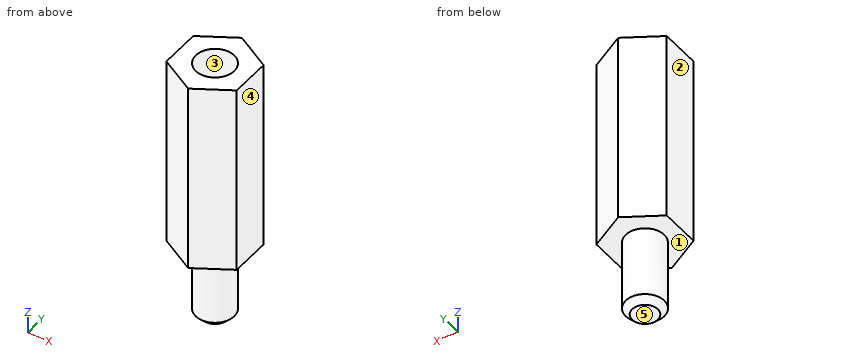
```python
from build123d import *

# Parameters (mm, degrees)
PAD014_DEPTH    = 15
SKETCH032_R     = 1.5
PAD013_DEPTH    = 6
SKETCH031_R     = 1.5
POCKET012_DEPTH = 8.5
CHAMFER011_SIZE = 1.5
CHAMFER012_SIZE = 0.5


with BuildPart() as part:
    # Sketch030 → Pad014 (new body)
    with BuildSketch(Plane.XY):
        Polygon((-2.75, -1.587713), (-2.75, 1.587713), (0, 3.175426), (2.75, 1.587713), (2.75, -1.587713), (0, -3.175426), align=None)
    extrude(amount=PAD014_DEPTH)

    # Sketch032 (on Face7 of Pad014) → Pad013 (new body)
    with BuildSketch(Plane(origin=(0, 0, 0), x_dir=(1, 0, 0), z_dir=(0, 0, -1))):
        Circle(SKETCH032_R)
    extrude(amount=PAD013_DEPTH)

    # Sketch031 (on Face5 of Pad013) → Pocket012 (cut)
    with BuildSketch(Plane.XY.offset(15)):
        Circle(SKETCH031_R)
    extrude(amount=-POCKET012_DEPTH, mode=Mode.SUBTRACT)

    # Chamfer011
    chamfer011_edges = [part.edges().sort_by_distance(p)[0] for p in [
        (-1.5, 0, 6.5),
    ]]
    chamfer(chamfer011_edges, length=CHAMFER011_SIZE)

    # Chamfer012
    chamfer012_edges = [part.edges().sort_by_distance(p)[0] for p in [
        (-1.5, 0, -6),
    ]]
    chamfer(chamfer012_edges, length=CHAMFER012_SIZE)


solid = part.part
```
Part model, mm, in its own coordinate system. Face numbers are marked on the shaded views. A direction names the side the tool comes from. Round coordinates to 2 decimals unless told otherwise and drop trailing zeros. Write each loop counter-clockwise with the first axis right and the second up, starting at its lowest first coordinate (ties: lowest second). Pieces come first, ordered by that corner, then holes. Notation, with made-up numbers: (31, 13.25) -> (77, 13.25) arc R32 cw to (77, 44.25) -> close; hole circle Ø4 at (43.5, -1.5). An arc over 180 degrees is marked (long way). Return JSON: item names as keys, results as strings. Group by question number.
Q1. Saw through at C-C on z = 11.5. Write the cut outline in (x, y), plus the area to 3 significant figures.
Q2. Saw through at D-D on y = 2.5. Write the cut outline in (x, z), plus the area to 3 significant figures.
Q3. Saw through at B-B on z = 0.25. Write the cut outline in (x, y), plus the area to 3 significant figures.
Q4. Saw through at A-A on z = 6.75. Write the cut outline in (x, y), plus the area to 3 significant figures.
Q5. Mould opens along X. For the marked faces 3, 4 and 5 say: pulls with the +X half, pulls with the -X half, needs draft (parallel to the pull), parting line crosses it, or undercut.
Q6. Which spindle directions (+Z, -Z, +X, -X, +Y, -Y) get a long thin tool onto all of the face, cutting with end or side? Do the marked faces 1 and 2. Say none if no direction does.
Q7. Probe L1, parallel to Y at x = 1, z = 9.5; L2, parallel to Z at x = -2, y = -1.25; L3, parallel to X at y = 1, z = -1. List the from-to ranges inside material, lowest first. Write a range as [from, to].
Q8. Pin check, flat tips, straight feed: pin 1 (1.5 mm diameter, centred on x = -0.5, z = 6, fed in from -Y); pin 2 (1.5 mm diameter, centred on x = -1.5, y = -1.5, fed in from -Z). Stop position of each tip, or through.
Answer:
{
 "1": {"outline": "(-2.75, -1.59) -> (0, -3.18) -> (2.75, -1.59) -> (2.75, 1.59) -> (0, 3.18) -> (-2.75, 1.59) -> close; hole circle Ø3 at (0, 0)", "area": "19.1 mm2"},
 "2": {"outline": "(-1.17, 0) -> (1.17, 0) -> (1.17, 15) -> (-1.17, 15) -> close", "area": "35.1 mm2"},
 "3": {"outline": "(-2.75, -1.59) -> (0, -3.18) -> (2.75, -1.59) -> (2.75, 1.59) -> (0, 3.18) -> (-2.75, 1.59) -> close", "area": "26.2 mm2"},
 "4": {"outline": "(-2.75, -1.59) -> (0, -3.18) -> (2.75, -1.59) -> (2.75, 1.59) -> (0, 3.18) -> (-2.75, 1.59) -> close; hole circle Ø0.5 at (0, 0)", "area": "26.0 mm2"},
 "5": {"face 3": "undercut", "face 4": "pulls with the +X half", "face 5": "needs draft"},
 "6": {"face 1": "-Z", "face 2": "+Z, -Z, -X, +Y, -Y"},
 "7": {"L1": "[-2.6, -1.12], [1.12, 2.6]", "L2": "[0, 15]", "L3": "[-1.12, 1.12]"},
 "8": {"pin 1": "y = -3.18", "pin 2": "z = -5.63"}
}
